For this review, use the dimensioned drawing (mm, ordinates from the lowest corner) and the shaded views. Coordinates: 2 decimals unless noted, no trailing zeros. Write each loop counter-clockwise with the first axis right and the second up, starting at its lowest first coordinate (ties: lowest second). Pieces come first, ordered by that corner, then holes. Notation, with made-up numbers: (22, 74) - (73, 74) arc R28 cw to (73, 100) - close; hole circle Ø5 at (-0.5, 10). An arc over 180 degrees is marked (long way). Use one line per item in the form item = value. Start each with the question number.
1) Insertion check: P1, Ø2, axis at x = 1, y = 3, coming from the -Z side; P2, Ø1.5, axis at x = 3.5, z = 17.5, coming from the +Y side. Each pin has a flat end and moves straight along its axis. Give the tip position at first contact, or say it passes through.
2) We need section C-C (y = 11.25). Give the boundary of the cut face in (x, z), plus the area to 4 significant figures.
3) For L1, parallel to Y at x = 1, z = 8.5; L2, parallel to X at y = 6, z = 8.25; L3, parallel to Y at x = 2.35, z = 14.25, list the stretches that pass through material, from the lowest coordinate up. Write a range as from..to.
4) We need section D-D (x = 3.1). Give the boundary of the cut face in (y, z).
5) We need section B-B (z = 13). Give the boundary of the cut face in (x, y), plus the area to 3 significant figures.
6) Mouldability with a two-part tool opening along X and no side actions: class the marked faces 1, 2, 3 and 4 as pulls with the +X half, pulls with the -X half, needs draft (parallel to the pull), parting line crosses it, or undercut.
7) We need section A-A (x = 1). Give the boundary of the cut face in (y, z).
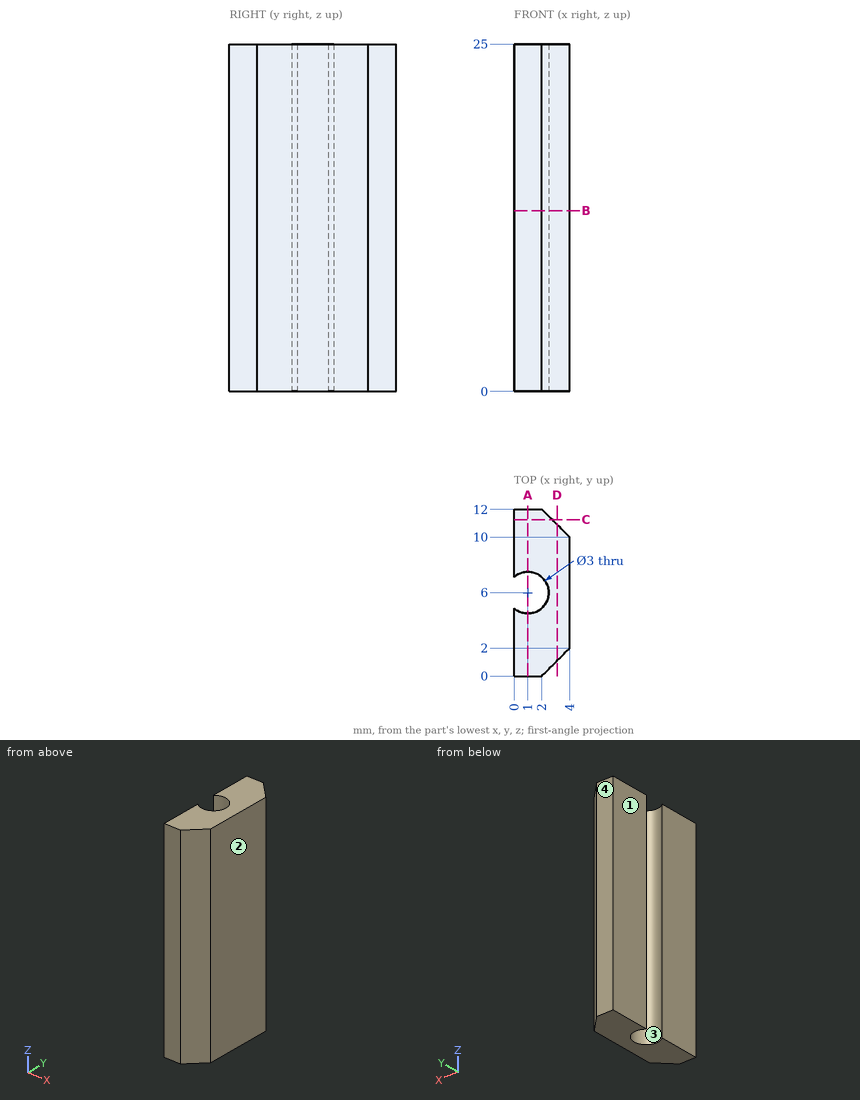
Determined:
q1.P1 = 0
q1.P2 = 11.25
q2.outline = (0, 0) - (2.75, 0) - (2.75, 25) - (0, 25) - close
q2.area = 68.75 mm²
q3.L1 = 0..4.5, 7.5..12
q3.L2 = 2.5..4
q3.L3 = 0.35..5.35, 6.65..11.65
q4.outline = (1.1, 0) - (10.9, 0) - (10.9, 25) - (1.1, 25) - close
q5.outline = (0, 0) - (2, 0) - (4, 2) - (4, 10) - (2, 12) - (0, 12) - (0, 7.12) arc R1.5 cw (long way) to (0, 4.88) - close
q5.area = 37.7 mm²
q6.face_1 = pulls with the -X half
q6.face_2 = pulls with the +X half
q6.face_3 = undercut
q6.face_4 = needs draft
q7.outline = (0, 0) - (4.5, 0) - (4.5, 25) - (0, 25) - close; (7.5, 0) - (12, 0) - (12, 25) - (7.5, 25) - close
